Read the model definition and answer for the solid it produces. Units are mm, in the model's axes. A direction names the side the tool comes from. Coordinates: 2 decimals unless noted, no trailing zeros. Write each loop counter-clockwise with the first axis right and the second up, starting at its lowest first coordinate (ties: lowest second). Pieces come first, ordered by that corner, then holes. Notation, with made-up numbers: (9, 88) - (24, 88) arc R19 cw to (24, 105) - close; hole circle Ø7 at (-34, 29). An arc over 180 degrees is marked (long way). Use a Markdown table: item, result.
from build123d import *

# Parameters (mm, degrees)
ESQUISSE1_W             = 28
ESQUISSE1_H             = 25.3
BOSS_EXTRU_1_DEPTH      = 28
BOSS_EXTRU_2_DEPTH      = 7.5
ESQUISSE3_R             = 3.25
ENL_V_MAT_EXTRU_1_DEPTH = 45.110344592
ESQUISSE4_W             = 0.8
ESQUISSE4_H             = 6.3
ESQUISSE4_W_2           = 6.3
ESQUISSE4_H_2           = 0.8
BOSS_EXTRU_3_DEPTH      = 10.2


with BuildPart() as part:
    # Esquisse1 → Boss.-Extru.1 (new body)
    with BuildSketch(Plane.XY):
        Rectangle(ESQUISSE1_W, ESQUISSE1_H)
    extrude(amount=BOSS_EXTRU_1_DEPTH)

    # Esquisse2 → Boss.-Extru.2 (add, symmetric)
    with BuildSketch(Plane(origin=(0, 0, 0), x_dir=(0, 0, -1), z_dir=(1, 0, 0))):
        Polygon((0, 12.65), (2, 17.44649219), (2, 29.15), (3.5, 29.15), (3.5, 17.44649219), (1.5, 12.65), (1.5, -3.073931528), (0, -3.073931528), align=None)
    extrude(amount=BOSS_EXTRU_2_DEPTH, both=True)

    # Esquisse3 → Enlèv. mat.-Extru.1 (cut, through all)
    with BuildSketch(Plane.XY.offset(-2)):
        with Locations((0, 23.15)):
            Circle(ESQUISSE3_R)
    extrude(amount=-ENL_V_MAT_EXTRU_1_DEPTH, mode=Mode.SUBTRACT)

    # Esquisse4 → Boss.-Extru.3 (add)
    with BuildSketch(Plane.XZ.offset(12.65)):
        with Locations((8.4, 16.8)):
            Rectangle(ESQUISSE4_W, ESQUISSE4_H)
        with Locations((0, 7.3)):
            Rectangle(ESQUISSE4_W, ESQUISSE4_H)
        with Locations((0, 25.2)):
            Rectangle(ESQUISSE4_W_2, ESQUISSE4_H_2)
        with Locations((-8.4, 16.8)):
            Rectangle(ESQUISSE4_W, ESQUISSE4_H)
        with Locations((0, 17.2)):
            Rectangle(ESQUISSE4_W_2, ESQUISSE4_H_2)
    extrude(amount=BOSS_EXTRU_3_DEPTH)


solid = part.part
(1) For faces 1 (the flat face through (-8, -18, 17)), 2 (the flat face through (8.8, -18, 17)), 3 (the flat face through (0, -18, 17.6)), 4 (the flat face through (3.4, 23.2, -2)), 5 (the flat face through (7.5, 13, -1)), determine the directions among +Z, -Z, +X, -X, +Y, -Y from which every point of the face is accessible in a straight line to the end or side of a thin tool.
Report:
| item | result |
|---|---|
| face 1 | +Z, -Z, -Y |
| face 2 | +Z, -Z, +X, -Y |
| face 3 | -Y |
| face 4 | +Z, +X, -X, +Y |
| face 5 | -Z, +X, +Y, -Y |
(2) The mould has two halves that part along X. Classify faces 6 (the flat face through (0, -18, 16.8)), 7 (the flat face through (-8.8, -18, 17)), 8 (the flat face through (0, 5, -1.5)): pulls with the +X half, pulls with the -X half, needs draft (parallel to the pull), parting line crosses it, or undercut.
Report:
| item | result |
|---|---|
| face 6 | undercut |
| face 7 | pulls with the -X half |
| face 8 | needs draft |
(3) A cutting plane is placed at B-B, the plane z = 19. Write down the section's boundary in (x, y), and give its area (3 significant figures).
Report:
| item | result |
|---|---|
| outline | (-14, -12.65) - (-8.8, -12.65) - (-8.8, -22.85) - (-8, -22.85) - (-8, -12.65) - (8, -12.65) - (8, -22.85) - (8.8, -22.85) - (8.8, -12.65) - (14, -12.65) - (14, 12.65) - (-14, 12.65) - close |
| area | 725 mm² |
(4) A cutting plane is placed at D-D, the plane y = 1.5. Write down the section's boundary in (x, z).
Report:
| item | result |
|---|---|
| outline | (-14, 0) - (-7.5, 0) - (-7.5, -1.5) - (7.5, -1.5) - (7.5, 0) - (14, 0) - (14, 28) - (-14, 28) - close |
(5) A cutting plane is placed at A-A, the plane y = 23.15. Write down the section's boundary in (x, z), and give its area (4 significant figures).
Report:
| item | result |
|---|---|
| outline | (-7.5, -3.5) - (-3.25, -3.5) - (-3.25, -2) - (-7.5, -2) - close; (3.25, -3.5) - (7.5, -3.5) - (7.5, -2) - (3.25, -2) - close |
| area | 12.75 mm² |
(6) Each of these flat-tipped pins is pushed along its axis until it touches: P1, Ø14, axis at x = 5.5, z = 17, coming from the +Y side; P2, Ø9.5, axis at x = 0.5, y = 24, coming from the +Z side; P3, Ø0.6, axis at x = 8.5, y = -18.5, coming from the +Z side. Where does it stop, or does it pass through?
Report:
| item | result |
|---|---|
| P1 | stops at y = 12.65 |
| P2 | stops at z = -2 |
| P3 | stops at z = 19.95 |
(7) A cutting plane is placed at C-C, the plane x = 5. Write down the section's boundary in (y, z), and give its area (3 significant figures).
Report:
| item | result |
|---|---|
| outline | (-12.65, 0) - (-3.07, 0) - (-3.07, -1.5) - (12.65, -1.5) - (17.45, -3.5) - (29.15, -3.5) - (29.15, -2) - (17.45, -2) - (12.65, 0) - (12.65, 28) - (-12.65, 28) - close |
| area | 757 mm² |
(8) Straight lines are drawn through the part: L1, parallel to X at y = 23, z = -3; L2, parallel to Z at x = -5.25, y = -2; L3, parallel to Z at x = 11.5, y = 0. For each, find the intervals that lie inside material, in ascending order.
Report:
| item | result |
|---|---|
| L1 | x = -7.5 to -3.25, 3.25 to 7.5 |
| L2 | z = -1.5 to 28 |
| L3 | z = 0 to 28 |
